```python
from build123d import *

# Parameters (mm, degrees)
SKETCH1_R                = 45
SKETCH1_R_2              = 10
BOSS_EXTRUDE1_DEPTH      = 20
BOSS_EXTRUDE2_DEPTH      = 15
BOSS_EXTRUDE2_DEPTH_BACK = 15


with BuildPart() as part:
    # Sketch1 → Boss-Extrude1 (new body)
    with BuildSketch(Plane(origin=(0, 0, 0), x_dir=(0, 0, -1), z_dir=(1, 0, 0))):
        Circle(SKETCH1_R)
        Circle(SKETCH1_R_2, mode=Mode.SUBTRACT)
    extrude(amount=BOSS_EXTRUDE1_DEPTH)

    # Sketch4 → Boss-Extrude2 (add, two sides: drawn at the far end of the back side and taken through both)
    with BuildSketch(Plane.XY.offset(-BOSS_EXTRUDE2_DEPTH_BACK)):
        Polygon((20, -15), (37.320508076, -45), (87.320508076, -45), (87.320508076, -35), (48.867513459, -35), (28.660254038, 0), (48.867513459, 35), (87.320508076, 35), (87.320508076, 45), (37.320508076, 45), (20, 15), align=None)
    extrude(amount=BOSS_EXTRUDE2_DEPTH + BOSS_EXTRUDE2_DEPTH_BACK)


solid = part.part
```
Model file for the job. Use its own axes, mm. A direction names the side the tool comes from. Coordinates: 2 decimals unless noted, no trailing zeros. Order: outer loops, then holes, each group sorted by start corner. A loop starts at its lowest first (then second) coordinate and runs counter-clockwise, first axis right, second up. Notation, with made-up numbers: M 24,6.5 L 52,6.5 A26 ccw 52,22.5 Z; hole C 28.25,8 d8. An arc over 180 degrees is marked long. Answer as CSV lines item,"result".
(1) Band-saw the part on A-A, the plane x = 56. List the corners of the cut face in (y, z).
Geometry says:
outline,"M -45,-15 L -35,-15 L -35,15 L -45,15 Z; M 35,-15 L 45,-15 L 45,15 L 35,15 Z"
(2) Pull direction X, two halves, no side cores. Call faces 4 (the flat face through (38.905, -17.745, -0.21)), 5 (the flat face through (63, 45, 0)), 6 (the flat face through (28.54, -29.79, -0.21)): +X half, -X half, draft (parallel to the pull), parting line (faces both ways), or undercut.
Geometry says:
face 4,"+X half"
face 5,"draft"
face 6,"undercut"
(3) Wall check: line 1 along Y through (x, z) = (15, 0); line 2 along Y through (x, z) = (83.5, 11.5); line 3 along Z through (x, y) = (48, 38). Give the ranges that are in metal, low to high.
Geometry says:
line 1,"y = -45 to -10, 10 to 45"
line 2,"y = -45 to -35, 35 to 45"
line 3,"z = -15 to 15"
(4) Band-saw the part on D-D, the plane x = 12. List the corners of the cut face in (y, z), then the cut area to 3 significant figures.
Geometry says:
outline,"C 0,0 d90; hole C 0,0 d20"
area,"6,050 mm2"
(5) 3-axis set-ups, long thin cutter, end or side, ignore diameter. For faces 1 (the flat face through (28.78, 30.21, -0.21)), 2 (the flat face through (31, 11, -15)), 3 (the flat face through (20, 1, -19)): which of +Z, -Z, +X, -X, +Y, -Y reach the whole face in a straight line?
Geometry says:
face 1,"+Z, -Z, +Y"
face 2,"-Z, +X, +Y, -Y"
face 3,"none"
(6) Band-saw the part on C-C, the plane z = 0. List the corners of the cut face in (x, y), then the cut area to 3 significant figures.
Geometry says:
outline,"M 0,-45 L 20,-45 L 20,-15 L 37.32,-45 L 87.32,-45 L 87.32,-35 L 48.87,-35 L 28.66,0 L 48.87,35 L 87.32,35 L 87.32,45 L 37.32,45 L 20,15 L 20,45 L 0,45 L 0,10 L 20,10 L 20,-10 L 0,-10 Z"
area,"3,540 mm2"
(7) Band-saw the part on B-B, the plane y = 33. List the corners of the cut face in (x, z), then the cut area to 3 significant figures.
Geometry says:
outline,"M 0,-30.59 L 20,-30.59 L 20,30.59 L 0,30.59 Z; M 30.39,-15 L 47.71,-15 L 47.71,15 L 30.39,15 Z"
area,"1,740 mm2"
(8) Flat gauge pins, fed straight in: pin 1 (1.5 mm diameter, centred on x = 42, y = -24.5, fed in from -Z); pin 2 (8 mm diameter, centred on x = 47, y = -17, fed in from +Z); pin 3 (6 mm diameter, centred on x = 50.5, y = 34, fed in from +Z); pin 4 (12 mm diameter, centred on x = 16, y = 13.5, fed in from -Z). Where does each tip first touch, or does it go through?
Geometry says:
pin 1,"stops at z = -15"
pin 2,"passes through"
pin 3,"stops at z = 15"
pin 4,"stops at z = -44.37"
